Can you work these out from the drawing? Everything is in mm from the part's minimum corner. Coordinates: 2 decimals unless noted, no trailing zeros. Write each loop counter-clockwise with the first axis right and the second up, starting at its lowest first coordinate (ties: lowest second). Pieces come first, ordered by that corner, then holes. Notation, with made-up numbers: M -1,15 L 9,15 A27 ccw 9,53 Z; hole C -8,23.25 d6. An arc over 180 degrees is marked long. Write item = value, one per line.
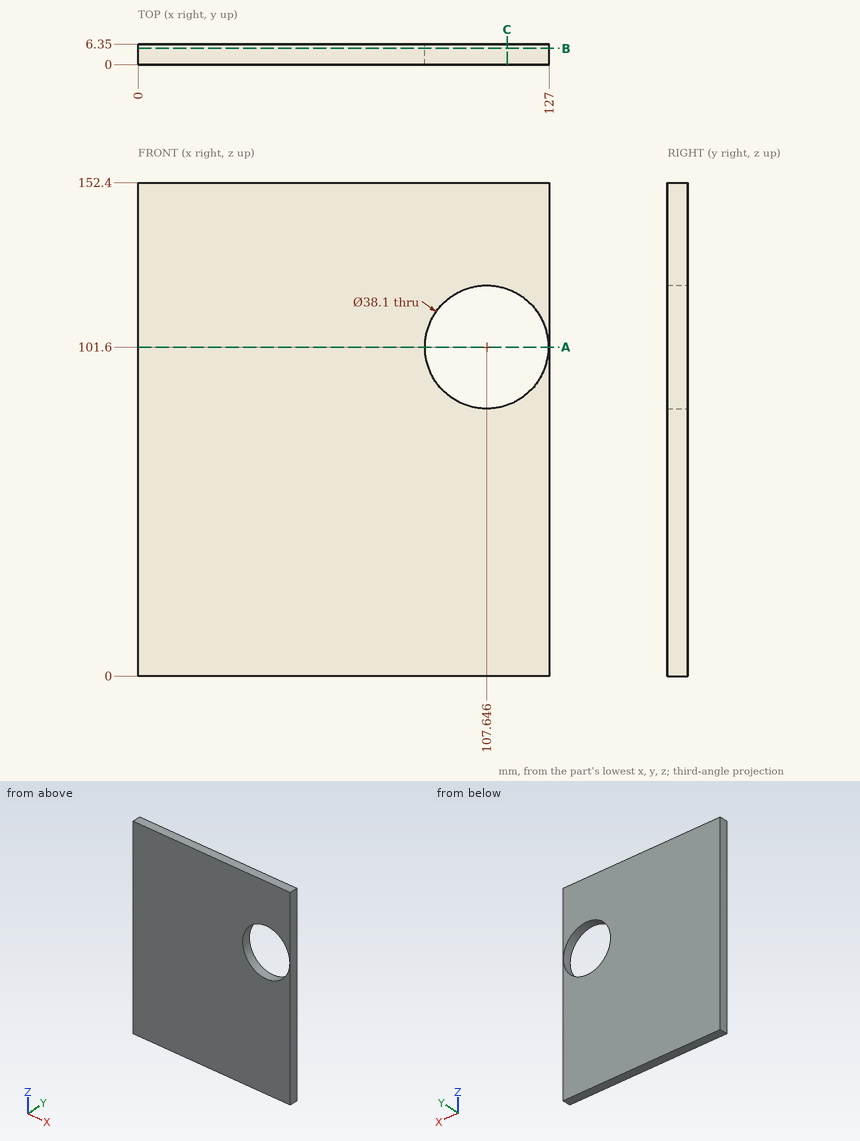
Item 1: Imagine slicing it at C-C (x = 114). Write out the boundary of the cut face in (y, z).
Numbers:
outline = M 0,0 L 6.35,0 L 6.35,83.64 L 0,83.64 Z; M 0,119.56 L 6.35,119.56 L 6.35,152.4 L 0,152.4 Z
Item 2: Imagine slicing it at B-B (y = 5). Write out the boundary of the cut face in (x, z), and give its area (3 significant figures).
Numbers:
outline = M 0,0 L 127,0 L 127,152.4 L 0,152.4 Z; hole C 107.65,101.6 d38.1
area = 18,200 mm²
Item 3: If I drill on line 1 along Z through (x, y) = (91, 1.5) (1 decimal); line 2 along Z through (x, y) = (118, 4); line 3 along X through (y, z) = (3.75, 87.5) (1 decimal), over which ranges is the centre line in solid material (lowest first)?
Numbers:
line_1 = 0 to 92.3, 110.9 to 152.4
line_2 = 0 to 85.61, 117.59 to 152.4
line_3 = 0 to 94.8, 120.5 to 127
Item 4: Imagine slicing it at A-A (z = 101.6). Write out the boundary of the cut face in (x, y).
Numbers:
outline = M 0,0 L 88.6,0 L 88.6,6.35 L 0,6.35 Z; M 126.7,0 L 127,0 L 127,6.35 L 126.7,6.35 Z
